Geometry: see drawing. Coordinates: mm, zero at the bounding-box minimum. Give positions to 0.01 mm unless a question says otherwise; leave off trailing zeros. Loops run counter-clockwise (first coordinate to the right, second up) from the corner with the lowest first, then second, coordinate; pieces in that order, holes last. Notation, with made-up numbers: M 61.5,8.5 L 105.5,8.5 A29 ccw 105.5,32.5 Z; hole C 22.5,-33.75 d1. An arc over 180 degrees is marked long. Put each result on its own line as item: value.
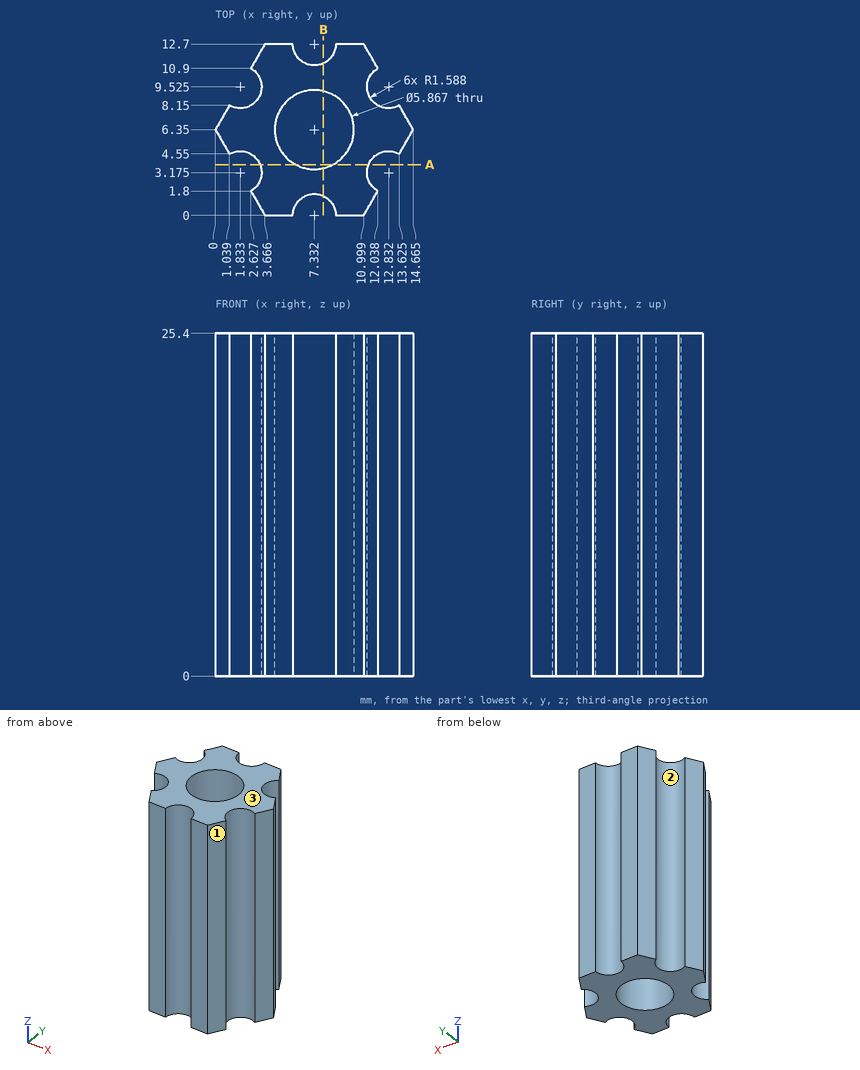
1. Contact query for a flat-ended pin moving along its axis: P1, Ø8, axis at x = 11, z = 21, coming from the -Y side. Output: stop coordinate, or through.
Found:
P1: y = 0
2. Section query B-B (x = 8). Output: boundary loops of the cut face in (y, z), plus the area to 3 significant figures.
Found:
outline: M 1.44,0 L 3.49,0 L 3.49,25.4 L 1.44,25.4 Z; M 9.21,0 L 11.26,0 L 11.26,25.4 L 9.21,25.4 Z
area: 104 mm^2
3. Section query A-A (y = 3.75). Output: boundary loops of the cut face in (x, z), plus the area to 3 significant figures.
Found:
outline: M 3.31,0 L 5.97,0 L 5.97,25.4 L 3.31,25.4 Z; M 8.69,0 L 11.35,0 L 11.35,25.4 L 8.69,25.4 Z
area: 135 mm^2
4. Material intervals for line 1 (Y direction, x = 2.75, z = 10) (1 decimal); line 2 (X direction, y = 5, z = 20.75) (1 decimal); line 3 (X direction, y = 6, z = 9.5) (1 decimal), sorted ascending. Write a range as from..to.
Found:
line 1: 1.6..1.9, 4.5..8.2, 10.8..11.1
line 2: 0.8..4.7, 9.9..13.9
line 3: 0.2..4.4, 10.2..14.5
5. Draft query along X for the marked faces 1, 2 and 3. Return one class per face: pulls with the +X half, pulls with the -X half, needs draft (parallel to the pull), parting line crosses it, or undercut.
Found:
face 1: pulls with the +X half
face 2: undercut
face 3: needs draft
